Read the model definition and answer for the solid it produces. Units are mm, in the model's axes. A direction names the side the tool comes from. Coordinates: 2 decimals unless noted, no trailing zeros. Order: outer loops, then holes, each group sorted by start corner. A loop starts at its lowest first (then second) coordinate and runs counter-clockwise, first axis right, second up. Notation, with made-up numbers: M -19.75,75.25 L -1.75,75.25 A26 ccw -1.75,112.25 Z; hole C 73,35 d4. An arc over 180 degrees is marked long. Use a Markdown table: item, result. Add a question column.
1) Find section B-B on y = 34. Write down the section's boundary in (x, z), plus the area to 3 significant figures.
2) The mould has two halves that part along X. Classify faces 3 (the face through (53.31, 52.06, 0.74)), 4 (the face through (-17.8, 41.71, 0.74)), 5 (the face through (-13, 68, 2.5)): released by +X, released by -X, zero draft, split by the parting line, or undercut.
3) Find section D-D on y = 47.5. Write down the section's boundary in (x, z).
4) For faces 1 (the face through (-19, 83, 2.5)), 2 (the face through (-13.38, 71.82, 1.99)), determine the directions among +Z, -Z, +X, -X, +Y, -Y from which every point of the face is accessible in a straight line to the end or side of a thin tool.
5) Find the intervals of material crossed by probe 1 along Z at (x, y) = (64, 82.5); probe 2 along X at (y, z) = (77, 2.45); probe 3 along X at (y, z) = (71, 2.1), in increasing order. Write a range as [from, to].
6) Each of these flat-tipped pins is pushed along its axis until it touches: pin 1 Ø3 at (x, y) = (-75.5, 68.5) entering from +Z; pin 2 Ø1 at (y, z) = (50, 0.5) entering from -X. Where does it stop, or does it pass through?
7) Find section C-C on z = 2.05. Write down the section's boundary in (x, y) (3 decimals).
8) Find section A-A on x = -13. Write down the section's boundary in (y, z).
from build123d import *

# Parameters (mm, degrees)
F1_DEPTH = 1.5
F2_R     = 0.625
F2_R_2   = 1.25
F2_R_3   = 3.75
F3_DEPTH = 1


with BuildPart() as f1:
    # F0 (on Top) → F1 (new body)
    with BuildSketch(Plane.XY):
        with BuildLine():
            Line((32.444928, 31.685156), (74.762845, 73.012102))
            ThreePointArc((74.762845, 73.012102), (-39.417843, 96.780595), (-104.5, 0))
            Line((-104.5, 0), (-45.35, 0))
            ThreePointArc((-45.35, 0), (-17.106212, 42), (32.444928, 31.685156))
        make_face()
    extrude(amount=F1_DEPTH)

    # F2 (on face) → F3 (join)
    with BuildSketch(Plane.XY.offset(1.5)):
        with BuildLine():
            ThreePointArc((-30.96232, 75.58918), (-30.884194, 75.612404), (-30.807747, 75.640671))
            Line((-30.807747, 75.640671), (-30.811752, 75.650505))
            Line((-30.811752, 75.650505), (-30.96232, 75.58918))
        make_face()
        with BuildLine():
            Line((-30.811752, 75.650505), (-30.807747, 75.640671))
            ThreePointArc((-30.807747, 75.640671), (-30.733305, 75.67386), (-30.661184, 75.71183))
            Line((-30.661184, 75.71183), (-30.811752, 75.650505))
        make_face()
        with BuildLine():
            Line((-30.96232, 75.58918), (-30.811752, 75.650505))
            Line((-30.811752, 75.650505), (-31.750758, 77.955996))
            ThreePointArc((-31.750758, 77.955996), (-32.465182, 76.403275), (-30.96232, 75.58918))
        make_face()
        with BuildLine():
            Line((-31.750758, 77.955996), (-30.811752, 75.650505))
            Line((-30.811752, 75.650505), (-30.661184, 75.71183))
            ThreePointArc((-30.661184, 75.71183), (-30.198724, 76.169878), (-30.029252, 76.798334))
            ThreePointArc((-30.029252, 76.798334), (-30.581715, 77.835609), (-31.750758, 77.955996))
        make_face()
        with BuildLine():
            ThreePointArc((-21.366645, 82.285112), (-21.337038, 82.208873), (-21.304953, 82.133643))
            Line((-21.304953, 82.133643), (-21.366645, 82.285112))
        make_face()
        with BuildLine():
            Line((-21.366645, 82.285112), (-21.304953, 82.133643))
            ThreePointArc((-21.304953, 82.133643), (-19.954269, 80.832328), (-18.078702, 80.836558))
            ThreePointArc((-18.078702, 80.836558), (-16.947162, 81.756808), (-16.521713, 83.151883))
            ThreePointArc((-16.521713, 83.151883), (-19.46198, 85.612811), (-21.366645, 82.285112))
        make_face()
        with Locations((-42.055275, 71.745973)):
            Circle(F2_R)
        with Locations((-36.397212, 57.854021)):
            Circle(F2_R_2)
        with Locations((-12.892144, 68.102269)):
            Circle(F2_R_3)
    extrude(amount=F3_DEPTH)


solid = f1.part
Check result:
| question | item | result |
|---|---|---|
| 1 | outline | M -98.81,0 L -30.01,0 L -30.01,1.5 L -98.81,1.5 Z; M 30.01,0 L 34.82,0 L 34.82,1.5 L 30.01,1.5 Z |
| 1 | area | 110 mm2 |
| 2 | face 3 | released by +X |
| 2 | face 4 | undercut |
| 2 | face 5 | zero draft |
| 3 | outline | M -93.08,0 L 48.64,0 L 48.64,1.5 L -93.08,1.5 Z |
| 4 | face 1 | +Z, +X, -X, +Y, -Y |
| 4 | face 2 | +Z |
| 5 | probe 1 | z = [0, 1.5] |
| 5 | probe 2 | x = [-32.51, -30.05] |
| 5 | probe 3 | x = [-15.27, -10.51] |
| 6 | pin 1 | stops at z = 1.5 |
| 6 | pin 2 | stops at x = -92.03 |
| 7 | outline | C -42.055,71.746 d1.25; C -36.397,57.854 d2.5; M -31.751,77.956 A1.25 ccw -30.962,75.589 A1.25 ccw -30.808,75.641 A1.25 ccw -30.661,75.712 A1.25 ccw -30.029,76.798 A1.25 ccw Z; M -21.367,82.285 A2.5 ccw -21.305,82.134 A2.5 ccw -18.079,80.837 A2.5 ccw -16.522,83.152 A2.5 ccw long Z; C -12.892,68.102 d7.5 |
| 8 | outline | M 43.45,0 L 103.69,0 L 103.69,1.5 L 71.85,1.5 L 71.85,2.5 L 64.35,2.5 L 64.35,1.5 L 43.45,1.5 Z |
